Check sheet for the modelled part. Datum: model origin and axes. Units: mm. Give positions to 0.01 mm unless a question says otherwise; leave off trailing zeros. Order: outer loops, then holes, each group sorted by start corner. A loop starts at its lowest first (then second) coordinate and runs counter-clockwise, first axis right, second up.
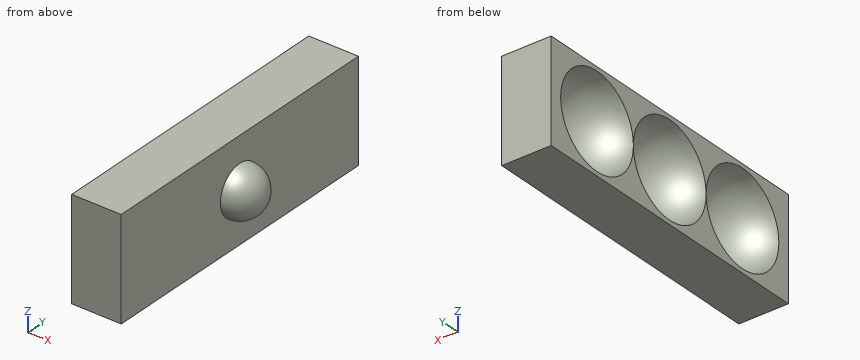
```python
from build123d import *

# Parameters (mm, degrees)
REVOLVE_1_ANGLE            = 180
EXTRUDE_1_DEPTH            = 10
EXTRUDE_1_DEPTH_BACK       = 10
SKETCH_5_W                 = 9.796885282
SKETCH_5_H                 = 60
PATTERN_LINEAR_1_COUNT     = 2
PATTERN_LINEAR_1_PITCH     = 18.4
PATTERN_LINEAR_1_COL_COUNT = 2
PATTERN_LINEAR_1_COL_PITCH = 18.4


with BuildPart() as part:
    # 草图1 → 旋转1 (revolve)
    with BuildSketch(Plane(origin=(0, 0, 0), x_dir=(0, 0, -1), z_dir=(1, 0, 0))):
        with BuildLine():
            Line((0, 4.9), (0, -4.9))
            ThreePointArc((0, -4.9), (4.9, 0), (0, 4.9))
        make_face()
    revolve(axis=Axis((0, 4.9, 0), (0, -1, 0)), revolution_arc=REVOLVE_1_ANGLE)

    # 草图5 → 凸台-拉伸1 (add, two sides: drawn at the far end of the back side and taken through both)
    with BuildSketch(Plane.XY.offset(-EXTRUDE_1_DEPTH_BACK)):
        with Locations((-4.898442641, 0)):
            Rectangle(SKETCH_5_W, SKETCH_5_H)
    extrude(amount=EXTRUDE_1_DEPTH + EXTRUDE_1_DEPTH_BACK)

    # 草图7 → 切除-旋转1 (revolve, cut)
    with BuildSketch(Plane.XY):
        with BuildLine():
            Line((-9.796885282, 9.2), (-9.796885282, -9.2))
            ThreePointArc((-9.796885282, -9.2), (-18.996885282, 0), (-9.796885282, 9.2))
        make_face()
    cut_revolve_1 = revolve(axis=Axis((-9.796885282, 9.2, 0), (0, -1, 0)), mode=Mode.SUBTRACT)

    # 阵列(线性)1: 切除-旋转1 ×2
    with Locations(*[(0, i * PATTERN_LINEAR_1_PITCH, 0) for i in range(1, PATTERN_LINEAR_1_COUNT)]):
        add(cut_revolve_1, mode=Mode.SUBTRACT)

    # 阵列(线性)1 col: 切除-旋转1 ×2
    with Locations(*[(0, -i * PATTERN_LINEAR_1_COL_PITCH, 0) for i in range(1, PATTERN_LINEAR_1_COL_COUNT)]):
        add(cut_revolve_1, mode=Mode.SUBTRACT)


solid = part.part
```
Q1. Sectioned sample at D-D, the plane z = -8.25. Record the cut outline in (x, y), plus the area to 3 significant figures.
Q2. Sectioned sample at C-C, the plane z = 1.75. Record the cut outline in (x, y), plus the area to 3 significant figures.
Q3. Material ranges on line 1 (Y direction, x = -7.5, z = 6); line 2 (Y direction, x = -5, z = 5); line 3 (Z direction, x = -4, y = 14.5), recorded low to high.
Q4. Sectioned sample at A-A, the plane x = -2.75. Record the cut outline in (y, z).
Q5. Sectioned sample at B-B, the plane y = -1. Record the cut outline in (x, z).
Q6. Go/stop test with flat-tipped pins: P1, Ø6, axis at y = -21.5, z = 1, coming from the -X side; P2, Ø3, axis at x = 3, z = -5, coming from the -Y side; P3, Ø3, axis at y = 19.5, z = -4.5, coming from the -X side. Record where each tip stops, or that it passes through.
Filled in:
1. outline: (-9.8, -30) - (0, -30) - (0, 30) - (-9.8, 30) - (-9.8, 22.47) arc R4.07 cw to (-9.8, 14.33) - (-9.8, 4.07) arc R4.07 cw to (-9.8, -4.07) - (-9.8, -14.33) arc R4.07 cw to (-9.8, -22.47) - close
1. area: 510 mm2
2. outline: (-9.8, -30) - (0, -30) - (0, -4.58) arc R4.58 ccw to (0, 4.58) - (0, 30) - (-9.8, 30) - (-9.8, 27.43) arc R9.03 cw to (-9.8, 9.37) - (-9.8, 9.03) arc R9.03 cw to (-9.8, -9.03) - (-9.8, -9.37) arc R9.03 cw to (-9.8, -27.43) - close
2. area: 236 mm2
3. line 1: y = -30 to -24.99, -11.81 to -6.59, 6.59 to 11.81, 24.99 to 30
3. line 2: y = -30 to -24.45, -12.35 to -6.05, 6.05 to 12.35, 24.45 to 30
3. line 3: z = -10 to -5.99, 5.99 to 10
4. outline: (-30, -10) - (30, -10) - (30, 10) - (-30, 10) - close; hole circle Ø11.83 at (-18.4, 0); hole circle Ø11.83 at (0, 0); hole circle Ø11.83 at (18.4, 0)
5. outline: (-9.8, -10) - (0, -10) - (0, -4.8) arc R4.8 ccw to (0, 4.8) - (0, 10) - (-9.8, 10) - (-9.8, 9.15) arc R9.15 cw to (-9.8, -9.15) - close
6. P1: stops at x = -3.05
6. P2: stops at y = -2.29
6. P3: stops at x = -2.94
